Verification items for the finished model (mm, model axes). A direction names the side the tool comes from. Coordinates: 2 decimals unless noted, no trailing zeros. Loops run counter-clockwise (first coordinate to the right, second up) from the corner with the lowest first, then second, coordinate; pieces in that order, holes last.
Q1. Sectioned sample at B-B (y = -6). Enter the section's corners in (x, z).
Q2. Go/stop test with flat-tipped pins: P1, Ø2, axis at y = -9.5, z = 8.5, coming from the -X side; P2, Ø1, axis at y = 10, z = 9, coming from the +X side; P3, Ø8, axis at x = 11, y = -26.5, coming from the -Z side; P4, Ø3, axis at x = -20, z = 10, coming from the -Y side. Record where each tip stops, or that it passes through.
Q3. Sectioned sample at C-C (z = 8.5). Enter the section's corners in (x, y), then the cut area to 3 significant figures.
Q4. Access from +Z, -Z, +X, -X, +Y, -Y to the whole of each face (thin tool, end or side, straight path). Record for faces 4 (the face through (-5.521, -10, 6)), 5 (the face through (-49.953, -5, 2)).
Q5. Sectioned sample at D-D (y = -22). Enter the section's corners in (x, z).
Q6. Mould release check, pull along Y, two halves, no side actions. Record for faces 1 (the face through (-1, -9.008, 6)), 2 (the face through (0, 29.374, 2)), 3 (the face through (-48.527, -4.171, 8.496)): +Y half, -Y half, draft (parallel to the pull), parting line (faces both ways), or undercut.
Q7. Material ranges on probe 1 along Y at (x, z) = (-3, 4.75); probe 2 along X at (y, z) = (-12, 10.75); probe 3 along Z at (x, y) = (0.5, -19.5), recorded low to high.
```python
from build123d import *

# Parameters (mm, degrees)
F0_W     = 101.8128246069
F0_H     = 68.0426731706
F1_DEPTH = 10
F2_R     = 5
F3_W     = 18.016605638
F3_H     = 28.1872702762
F4_DEPTH = 2.5
F5_W     = 10.1706655696
F5_H     = 2.0341333002
F5_H_2   = 2.3247234058
F6_DEPTH = 25
F7_R     = 2.49999


# Not quite as in the source:
# - a fillet or chamfer is up to 0.001 mm smaller than in the source, because OpenCascade refuses the exact size


with BuildPart() as f1:
    # F0 (on Top) → F1 (new body)
    with BuildSketch(Plane.XY):
        with Locations((0.9539090097, -4.6469829977)):
            Rectangle(F0_W, F0_H)
    extrude(amount=F1_DEPTH)

    # F2
    f2_edges = [f1.edges().sort_by_distance(p)[0] for p in [
        (-49.952503, -4.646983, 10),
        (0.953909, 29.374354, 10),
        (0.953909, -38.66832, 10),
        (51.860321, -4.646983, 10),
    ]]
    fillet(f2_edges, radius=F2_R)

    # F3 (on face) → F4 (join)
    with BuildSketch(Plane.XY.offset(10)):
        with Locations((-0.5811811425, -5.3759221919)):
            Rectangle(F3_W, F3_H)
    extrude(amount=F4_DEPTH)

    # F5 (on face) → F6 (cut)
    with BuildSketch(Plane.XY.offset(12.5)):
        with Locations((-0.435885042, -10.0253690034)):
            Rectangle(F5_W, F5_H)
        with Locations((-0.435885042, -1.1623617029)):
            Rectangle(F5_W, F5_H_2)
    extrude(amount=-F6_DEPTH, mode=Mode.SUBTRACT)

    # F7 (radius 2.5 in the source; OpenCascade refuses exactly that, so slightly less here)
    f7_edges = [f1.edges().sort_by_distance(p)[0] for p in [
        (-0.581181, -19.469557, 12.5),
        (-0.581181, 8.717713, 12.5),
    ]]
    fillet(f7_edges, radius=F7_R)


solid = f1.part
```
Geometry check:
1. outline: (-49.95, 0) - (51.86, 0) - (51.86, 5) arc R5 ccw to (46.86, 10) - (8.43, 10) - (8.43, 12.5) - (-9.59, 12.5) - (-9.59, 10) - (-44.95, 10) arc R5 ccw to (-49.95, 5) - close
2. P1: stops at x = -49.28
2. P2: stops at x = 50.43
2. P3: stops at z = 0
2. P4: stops at y = -37.24
3. outline: (-48.52, -37.24) - (50.43, -37.24) - (50.43, 27.95) - (-48.52, 27.95) - close; hole (-5.52, -11.04) - (4.65, -11.04) - (4.65, -9.01) - (-5.52, -9.01) - close; hole (-5.52, -2.32) - (4.65, -2.32) - (4.65, 0) - (-5.52, 0) - close
3. area: 6,410 mm2
4. face 4: +Z, -Z
4. face 5: +Z, -Z, -X, +Y, -Y
5. outline: (-49.95, 0) - (51.86, 0) - (51.86, 5) arc R5 ccw to (46.86, 10) - (-44.95, 10) arc R5 ccw to (-49.95, 5) - close
6. face 1: undercut
6. face 2: +Y half
6. face 3: draft
7. probe 1: y = -38.67 to -11.04, -9.01 to -2.32, 0 to 29.37
7. probe 2: x = -9.59 to 8.43
7. probe 3: z = 0 to 10
